The model under review builds one solid part; all positions refer to its coordinate system, in mm. Face numbers are marked on the shaded views. A direction names the side the tool comes from. Give positions to 0.01 mm unless a question says otherwise; leave off trailing zeros. Order: outer loops, then holes, each group sorted by start corner. A loop starts at its lowest first (then second) coordinate and runs counter-clockwise, first axis right, second up.
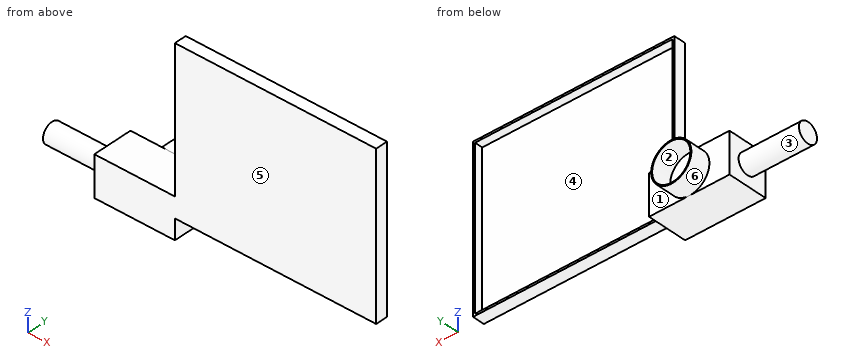
```python
from build123d import *

# Parameters (mm, degrees)
SKETCH1_R           = 25
BOSS_EXTRUDE1_DEPTH = 150
SKETCH2_W           = 100
SKETCH2_H           = 100
BOSS_EXTRUDE2_DEPTH = 200
SKETCH3_R           = 50
SKETCH3_R_2         = 47.5
BOSS_EXTRUDE3_DEPTH = 50
SKETCH4_W           = 500
SKETCH4_H           = 400
SKETCH4_W_2         = 490
SKETCH4_H_2         = 390
BOSS_EXTRUDE4_DEPTH = 30
SKETCH5_W           = 490
SKETCH5_H           = 390
BOSS_EXTRUDE5_DEPTH = 10


with BuildPart() as part:
    # Sketch1 → Boss-Extrude1 (new body)
    with BuildSketch(Plane(origin=(0, 0, 0), x_dir=(0, 0, -1), z_dir=(1, 0, 0))):
        Circle(SKETCH1_R)
    extrude(amount=BOSS_EXTRUDE1_DEPTH)

    # Sketch2 → Boss-Extrude2 (add)
    with BuildSketch(Plane(origin=(150, 0, 0), x_dir=(0, 0, -1), z_dir=(1, 0, 0))):
        Rectangle(SKETCH2_W, SKETCH2_H)
    extrude(amount=BOSS_EXTRUDE2_DEPTH)

    # Sketch3 → Boss-Extrude3 (add)
    with BuildSketch(Plane(origin=(0, 50, 0), x_dir=(1, 0, 0), z_dir=(0, 1, 0))):
        with Locations((250, 0)):
            Circle(SKETCH3_R)
        with Locations((250, 0)):
            Circle(SKETCH3_R_2, mode=Mode.SUBTRACT)
    extrude(amount=BOSS_EXTRUDE3_DEPTH)

    # Sketch4 → Boss-Extrude4 (add)
    with BuildSketch(Plane(origin=(0, -50, 0), x_dir=(1, 0, 0), z_dir=(0, 1, 0))):
        with Locations((600, -200)):
            Rectangle(SKETCH4_W, SKETCH4_H)
        with Locations((600, -200)):
            Rectangle(SKETCH4_W_2, SKETCH4_H_2, mode=Mode.SUBTRACT)
    extrude(amount=BOSS_EXTRUDE4_DEPTH)

    # Sketch5 → Boss-Extrude5 (add)
    with BuildSketch(Plane.XZ.offset(50)):
        with Locations((600, 200)):
            Rectangle(SKETCH5_W, SKETCH5_H)
    extrude(amount=-BOSS_EXTRUDE5_DEPTH)


solid = part.part
```
1. Take a section at D-D (x = 137.5). Write out the cut boundary in (y, z).
2. Take a section at C-C (y = 71.5). Write out the cut boundary in (x, z), and give its area (3 significant figures).
3. To check wall thickness, follow line 1 (X direction, y = 62, z = 0); line 2 (X direction, y = -36.5, z = 223); line 3 (Z direction, x = 492.5, y = -30). State the ranges of each line that lie inside material, in increasing order.
4. For the marked faces 1, 2 and 3, list the 3-axis set-ups (+Z, -Z, +X, -X, +Y, -Y) from which the entire face can be reached by the end or side of a thin tool; tool diameter is ignored.
5. Take a section at A-A (y = 0). Write out the cut boundary in (x, z), and give its area (3 significant figures).
6. Draft analysis for pull direction X (two halves, no side actions). For the marked faces 4, 5 and 6, state which applies: pulls with the +X half, pulls with the -X half, needs draft (parallel to the pull), parting line crosses it, or undercut.
7. Take a section at B-B (x = 767). Write out the cut boundary in (y, z).
8. Insertion check: pin 1 (9 mm diameter, centred on x = 686.5, y = -29, fed in from -Z); pin 2 (1 mm diameter, centred on x = 237, y = -4.5, fed in from +Z); pin 3 (6 mm diameter, centred on y = -28.5, z = 133.5, fed in from -X). Each pin has a flat end and moves straight along its axis. Give the tip position at first contact, or say it passes through.
Answer:
1. outline: circle Ø50 at (0, 0)
2. outline: circle Ø100 at (250, 0); hole circle Ø95 at (250, 0)
2. area: 766 mm2
3. line 1: x = 200 to 202.5, 297.5 to 300
3. line 2: x = 350 to 355, 845 to 850
3. line 3: z = 0 to 5, 395 to 400
4. face 1: +X, +Y
4. face 2: +Y
4. face 3: -X
5. outline: (0, -25) - (150, -25) - (150, -50) - (350, -50) - (350, 50) - (150, 50) - (150, 25) - (0, 25) - close
5. area: 27,500 mm2
6. face 4: undercut
6. face 5: needs draft
6. face 6: parting line crosses it
7. outline: (-50, 0) - (-20, 0) - (-20, 5) - (-40, 5) - (-40, 395) - (-20, 395) - (-20, 400) - (-50, 400) - close
8. pin 1: stops at z = 0
8. pin 2: stops at z = 50
8. pin 3: stops at x = 350
